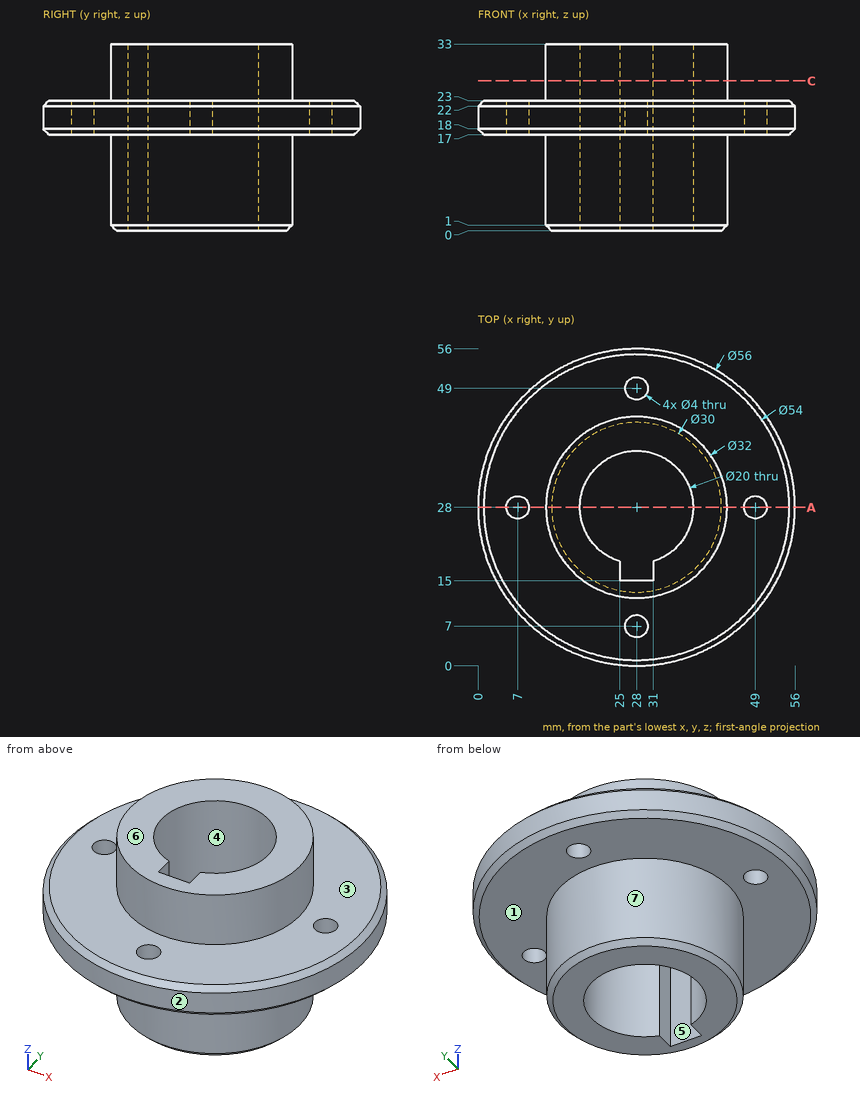
Print and shaded views of the part. All mm, measured from the part's lowest x, y and z. A direction names the side the tool comes from. Coordinates: 2 decimals unless noted, no trailing zeros. Order: outer loops, then holes, each group sorted by start corner. A loop starts at its lowest first (then second) coordinate and runs counter-clockwise, first axis right, second up.
(1) Probe L1, parallel to Y at x = 23, z = 10.5; L2, parallel to Z at x = 46, y = 10; L3, parallel to X at y = 7, z = 21.35. List the from-to ranges inside material, lowest first.
Check sheet entries:
L1: y = 12.8 to 19.34, 36.66 to 43.2
L2: z = 17 to 23
L3: x = 9.48 to 26, 30 to 46.52
(2) Pull direction X, two halves, no side cores. Call the marked faces 4, 5, 6 and 7: pulls with the +X half, pulls with the -X half, needs draft (parallel to the pull), parting line crosses it, or undercut.
Check sheet entries:
face 4: undercut
face 5: undercut
face 6: needs draft
face 7: parting line crosses it
(3) Pin check, flat tips, straight feed: pin 1 Ø3.5 at (x, y) = (28, 7) entering from -Z; pin 2 Ø12 at (x, z) = (30.5, 8) entering from -Y; pin 3 Ø12 at (y, z) = (23, 25.5) entering from -X; pin 4 Ø2 at (x, z) = (14, 28) entering from +Y. Stop position of each tip, or through.
Check sheet entries:
pin 1: passes through
pin 2: stops at y = 12
pin 3: stops at x = 0
pin 4: stops at y = 37.33
(4) Tool access for the marked faces 1, 2 and 3: list every direction of +Z, -Z, +X, -X, +Y, -Y with a clear straight run to the whole face (end or side of a thin tool).
Check sheet entries:
face 1: -Z
face 2: +Z, -Z
face 3: +Z
(5) Slice it at A-A, the plane y = 28. State how many separate pieces and enclosed holes the cut face has, and give its area (3 significant figures).
Check sheet entries:
separate pieces: 4
enclosed holes: 0
area: 489 mm2
(6) Slice it at C-C, the plane z = 26.5. Write the cut outline in (x, y).
Check sheet entries:
outline: circle Ø32 at (28, 28); hole (25, 15) - (31, 15) - (31, 18.46) arc R10 ccw (long way) to (25, 18.46) - close
